Job drawing, mm, ordinate dimensions from the low corner. One solid piece. Round coordinates to 2 decimals unless told otherwise and drop trailing zeros. Loops run counter-clockwise (first coordinate to the right, second up) from the corner with the lowest first, then second, coordinate; pieces in that order, holes last. Notation, with made-up numbers: M -2.75,59 L 23.25,59 A14 cw 23.25,72 Z; hole C 85,42.5 d7. An arc over 180 degrees is marked long. Put each result on its own line as item: value. Start each with the question number.
1) Slice it at B-B on z = 54. Give the cut face in (x, y), then the cut area to 3 significant figures.
2) Slice it at A-A on y = 1.8. Give the cut face in (x, z), then the cut area to 3 significant figures.
3) Probe line 1 along X through (y, z) = (2.15, 62.5); line 2 along Z through (x, y) = (14.5, 2.6); line 3 along X through (y, z) = (1.1, 46.5). List the from-to ranges inside material, lowest first.
4) Slice it at D-D on z = 5. Give the cut face in (x, y), then the cut area to 3 significant figures.
5) Slice it at C-C on x = 167.5. Give the cut face in (y, z), then the cut area to 3 significant figures.
6) Drop a flat-ended pin along its axis: pin 1 Ø0.9 at (x, y) = (89, 1) entering from +Z. Give the stop position or say it passes through.
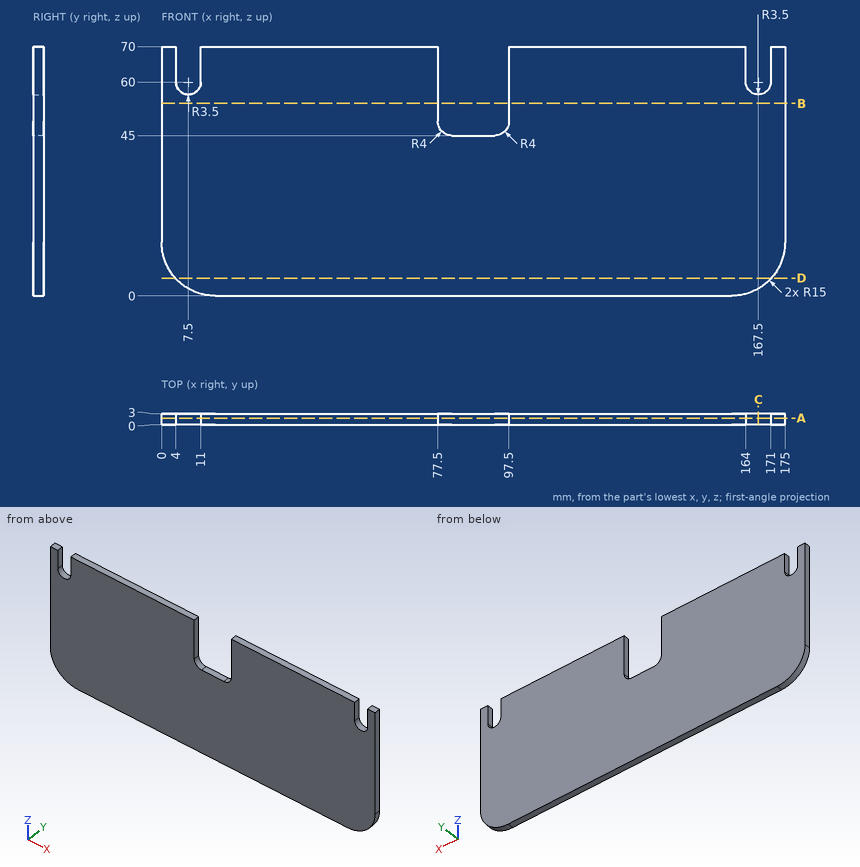
Recorded:
1. outline: M 0,0 L 77.5,0 L 77.5,3 L 0,3 Z; M 97.5,0 L 175,0 L 175,3 L 97.5,3 Z
1. area: 465 mm2
2. outline: M 0,15 A15 ccw 15,0 L 160,0 A15 ccw 175,15 L 175,70 L 171,70 L 171,60 A3.5 cw 164,60 L 164,70 L 97.5,70 L 97.5,49 A4 cw 93.5,45 L 81.5,45 A4 cw 77.5,49 L 77.5,70 L 11,70 L 11,60 A3.5 cw 4,60 L 4,70 L 0,70 Z
2. area: 11,500 mm2
3. line 1: x = 0 to 4, 11 to 77.5, 97.5 to 164, 171 to 175
3. line 2: z = 0.01 to 70
3. line 3: x = 0 to 78.38, 96.62 to 175
4. outline: M 3.82,0 L 171.18,0 L 171.18,3 L 3.82,3 Z
4. area: 502 mm2
5. outline: M 0,2.01 L 3,2.01 L 3,56.5 L 0,56.5 Z
5. area: 163 mm2
6. pin 1: stops at z = 45
